Can you work these out from the model? Positions are in its coordinate system, mm. A direction names the side the tool comes from. Coordinates: 2 decimals unless noted, no trailing zeros. Order: outer loops, then holes, each group sorted by start corner. A loop starts at its lowest first (then second) coordinate and runs counter-clockwise, first axis right, second up. Notation, with made-up numbers: (18, 5) -> (39, 5) arc R27 cw to (39, 32) -> close; hole circle Ø7 at (-3.75, 75.25). An arc over 180 degrees is marked (long way). Answer in a Markdown table with one row per item.
Autodesk Inventor part; units mm, degrees
ref_plane "YZ Plane" through (0, 0, 0) normal (1, 0, 0) x (0, 1, 0)
ref_plane "XZ Plane" through (0, 0, 0) normal (0, 1, 0) x (-1, 0, 0)
ref_plane "XY Plane" through (0, 0, 0) normal (0, 0, 1) x (1, 0, 0)
sketch "草圖1" plane through (0, 0, 0) normal (0, 0, 1) x (1, 0, 0)
  line L0 (35, -20) -> (-35, -20)
  line L1 (-35, -20) -> (-35, 20)
  line L2 (-35, 20) -> (35, 20)
  line L3 (35, 20) -> (35, -20)
  line L4 (35, -20) -> (-35, 20) construction
  line L5 (-35, -20) -> (35, 20) construction
  point P0 (0, 0)
  dimension "d0" = 70
  dimension "d1" = 40
extrude "擠出1" add sketch "草圖1" along normal blind 10
sketch "草圖2" plane through (0, 0, 10) normal (0, 0, 1) x (1, 0, 0)
  line L0 (35, 20) -> (-35, 20)
  line L1 (-35, 20) -> (5, 20)
  line L2 (5, 20) -> (5, 0)
  line L3 (5, 0) -> (-35, 0)
  line L4 (-35, 0) -> (-35, 20)
  line L5 (35, 20) -> (15, 20)
  line L6 (15, 20) -> (15, 10)
  line L7 (15, 10) -> (35, 10)
  line L8 (35, 10) -> (35, 20)
  point P0 (0, 0)
  point P1 (5, 20)
  dimension "d4" = 20
  dimension "d5" = 10
  dimension "d6" = 40
  dimension "d7" = 20
extrude "擠出2" add sketch "草圖2" along normal blind 30
sketch "草圖3" plane through (-35, 0, 10) normal (0, -1, 0) x (1, 0, 0)
  circle A0 centre (20, 30) radius 10
  line L0 (0, 0) -> (0, 30)
  line L1 (0, 0) -> (70, 0)
  point P0 (35, -10)
  dimension "d14" = 20
  dimension "d15" = 20
  dimension "d16" = 30
extrude "擠出3" cut sketch "草圖3" against normal blind 30
sketch "草圖4" plane through (5, 0, 10) normal (1, 0, 0) x (0, 0, -1)
  line L0 (-30, 20) -> (-30, 0)
  line L1 (-30, 0) -> (-0.078, 0)
  line L2 (-0.078, 0) -> (-0.078, 20)
  line L3 (-0.078, 20) -> (-30, 20)
  line L4 (-30, 20) -> (-30, 0)
  point P0 (10, 0)
loft "斷面混成2" add section 1 edges at (15, 15, 10) (15, 10, 25) (15, 15, 40) (15, 20, 25) section 2 edges at (5, 10, 10) (5, 20, 25) (5, 10, 40) (5, 0, 25)
properties part number "件28"
(1) Suppose I cut it at A-A (z = 37.5). Please give me the cut outline in (x, y).
Response values:
| item | result |
|---|---|
| outline | (-35, 0) -> (-24.68, 0) -> (-24.68, 20) -> (-35, 20) -> close; (-5.32, 0) -> (5, 0) -> (15, 10) -> (35, 10) -> (35, 20) -> (-5.32, 20) -> close |
(2) Suppose I cut it at B-B (y = 1.5). Please give me the cut outline in (x, z), and give its area (3 significant figures).
Response values:
| item | result |
|---|---|
| outline | (-35, 0) -> (35, 0) -> (35, 10) -> (6.5, 10) -> (6.5, 40) -> (-5, 40) arc R10 cw to (-25, 40) -> (-35, 40) -> close |
| area | 1,790 mm2 |
(3) Will these pins go through, and if not, where does the flat tip stop? pin 1 Ø15 at (x, z) = (-9, 19.5) entering from -Y; pin 2 Ø4 at (x, y) = (-17, 0) entering from +Z; pin 3 Ø4 at (x, z) = (14, 19.5) entering from -Y.
Response values:
| item | result |
|---|---|
| pin 1 | y = 0 |
| pin 2 | z = 30.83 |
| pin 3 | y = 7 |
(4) On a 3-axis mill with a long thin cutter (end or side, diameter ignored), from which of +Z, -Z, +X, -X, +Y, -Y can I reach the whole of each face in a straight line? I mean faces 1 (the flat face through (-15, 0, 21)), 2 (the flat face through (10, 5, 25)), 3 (the flat face through (0, 0, 0)). Say none if no direction works.
Response values:
| item | result |
|---|---|
| face 1 | +Z, +X, -X, -Y |
| face 2 | +Z, +X, -Y |
| face 3 | -Z, +X, -X, +Y, -Y |
(5) We'd pull the mould along X, two halves only. Please class faces 4 (the flat face through (-30, 10, 40)), 5 (the flat face through (35, 9, 6)), 6 (the cylindrical face through (-15, 10, 30)): +X half, -X half, draft (parallel to the pull), parting line (faces both ways), or undercut.
Response values:
| item | result |
|---|---|
| face 4 | draft |
| face 5 | +X half |
| face 6 | undercut |
(6) Suppose I cut it at D-D (x = 28.5). Please give me the cut outline in (y, z).
Response values:
| item | result |
|---|---|
| outline | (-20, 0) -> (20, 0) -> (20, 40) -> (10, 40) -> (10, 10) -> (-20, 10) -> close |
(7) Suppose I cut it at C-C (x = -9). Please give me the cut outline in (y, z), and give its area (3 significant figures).
Response values:
| item | result |
|---|---|
| outline | (-20, 0) -> (20, 0) -> (20, 32) -> (0, 32) -> (0, 10) -> (-20, 10) -> close |
| area | 840 mm2 |
(8) I need wall thicknesses on line 1 (Z direction, x = -26, y = -12); line 2 (Y direction, x = 29.5, z = 33); line 3 (X direction, y = 17, z = 35.5). Which ranges of each line are inside material? Lowest first, please. Write a range as [from, to].
Response values:
| item | result |
|---|---|
| line 1 | [0, 10] |
| line 2 | [10, 20] |
| line 3 | [-35, -23.93], [-6.07, 35] |
